Source: CAD feature listing. Evaluate the final solid. Frame: model axes, mm. Give positions to 0.01 mm unless a question says otherwise; leave off trailing zeros. Loops run counter-clockwise (first coordinate to the right, second up) from the corner with the lowest first, then second, coordinate; pieces in that order, holes last. Notation, with made-up numbers: M -35.75,11 L 8.25,11 A25 cw 8.25,47 Z; hole C 54.5,42 d10. An arc over 180 degrees is marked long. Answer in a Markdown table with one row per item.
```python
from build123d import *

# Parameters (mm, degrees)
AUFSATZ_LINEAR_AUSTRAGEN1_DEPTH = 2
AUFSATZ_LINEAR_START            = 2
AUFSATZ_LINEAR_AUSTRAGEN2_DEPTH = 2
SCHNITT_LINEAR_START            = -34
SCHNITT_LINEAR_AUSTRAGEN1_DEPTH = 34
VERRUNDUNG2_START               = 6.1999999
VERRUNDUNG2_3_DEPTH             = 116.6000001


with BuildPart() as part:
    # Skizze1 → Aufsatz-Linear austragen1 (new body)
    with BuildSketch(Plane(origin=(0, 0, 0), x_dir=(1, 0, 0), z_dir=(0, 1, 0))):
        with BuildLine():
            Line((3, 0), (249, 0))
            ThreePointArc((249, 0), (251.121320344, -0.878679656), (252, -3))
            Line((252, -3), (252, -126))
            ThreePointArc((252, -126), (251.121320344, -128.121320344), (249, -129))
            Line((249, -129), (3, -129))
            ThreePointArc((3, -129), (0.878679656, -128.121320344), (0, -126))
            Line((0, -126), (0, -3))
            ThreePointArc((0, -3), (0.878679656, -0.878679656), (3, 0))
        make_face()
        with BuildLine():
            Line((6.2, -3.2), (245.8, -3.2))
            ThreePointArc((245.8, -3.2), (247.921320344, -4.078679656), (248.8, -6.2))
            Line((248.8, -6.2), (248.8, -122.8))
            ThreePointArc((248.8, -122.8), (247.921320344, -124.921320344), (245.8, -125.8))
            Line((245.8, -125.8), (6.2, -125.8))
            ThreePointArc((6.2, -125.8), (4.078679656, -124.921320344), (3.2, -122.8))
            Line((3.2, -122.8), (3.2, -6.2))
            ThreePointArc((3.2, -6.2), (4.078679656, -4.078679656), (6.2, -3.2))
        make_face(mode=Mode.SUBTRACT)
    extrude(amount=AUFSATZ_LINEAR_AUSTRAGEN1_DEPTH)

    # Skizze2 → Aufsatz-Linear austragen2 (add)
    with BuildSketch(Plane.XZ.offset(AUFSATZ_LINEAR_START)):
        with BuildLine():
            Line((6.2, 126.8), (245.8, 126.8))
            ThreePointArc((245.8, 126.8), (248.628427125, 125.628427125), (249.8, 122.8))
            Line((249.8, 122.8), (249.8, 6.2))
            ThreePointArc((249.8, 6.2), (248.628427125, 3.371572875), (245.8, 2.2))
            Line((245.8, 2.2), (6.2, 2.2))
            ThreePointArc((6.2, 2.2), (3.371572875, 3.371572875), (2.2, 6.2))
            Line((2.2, 6.2), (2.2, 122.8))
            ThreePointArc((2.2, 122.8), (3.371572875, 125.628427125), (6.2, 126.8))
        make_face()
        with BuildLine():
            Line((248.8, 122.8), (248.8, 6.2))
            ThreePointArc((248.8, 6.2), (247.921320344, 4.078679656), (245.8, 3.2))
            Line((245.8, 3.2), (6.2, 3.2))
            ThreePointArc((6.2, 3.2), (4.078679656, 4.078679656), (3.2, 6.2))
            Line((3.2, 6.2), (3.2, 122.8))
            ThreePointArc((3.2, 122.8), (4.078679656, 124.921320344), (6.2, 125.8))
            Line((6.2, 125.8), (245.8, 125.8))
            ThreePointArc((245.8, 125.8), (247.921320344, 124.921320344), (248.8, 122.8))
        make_face(mode=Mode.SUBTRACT)
    extrude(amount=-AUFSATZ_LINEAR_AUSTRAGEN2_DEPTH)

    # Skizze3 → Schnitt-Linear austragen1 (cut)
    with BuildSketch(Plane(origin=(0, 2, 0), x_dir=(1, 0, 0), z_dir=(0, 1, 0)).offset(SCHNITT_LINEAR_START)):
        with BuildLine():
            Line((249, 0), (3, 0))
            ThreePointArc((3, 0), (0.878679656, -0.878679656), (0, -3))
            Line((0, -3), (0, -126))
            ThreePointArc((0, -126), (0.878679656, -128.121320344), (3, -129))
            Line((3, -129), (249, -129))
            ThreePointArc((249, -129), (251.121320344, -128.121320344), (252, -126))
            Line((252, -126), (252, -3))
            ThreePointArc((252, -3), (251.121320344, -0.878679656), (249, 0))
        make_face()
        with BuildLine():
            Line((249, -0.2), (3, -0.2))
            ThreePointArc((3, -0.2), (1.020101013, -1.020101013), (0.2, -3))
            Line((0.2, -3), (0.2, -126))
            ThreePointArc((0.2, -126), (1.020101013, -127.979898987), (3, -128.8))
            Line((3, -128.8), (249, -128.8))
            ThreePointArc((249, -128.8), (250.979898987, -127.979898987), (251.8, -126))
            Line((251.8, -126), (251.8, -3))
            ThreePointArc((251.8, -3), (250.979898987, -1.020101013), (249, -0.2))
        make_face(mode=Mode.SUBTRACT)
    extrude(amount=SCHNITT_LINEAR_AUSTRAGEN1_DEPTH, mode=Mode.SUBTRACT)

    # Verrundung2: read off the stored shape, not the designer's step
    # Verrundung2 outline → Verrundung2 (revolve, cut)
    with BuildSketch(Plane(origin=(245.8, 0, 122.8), x_dir=(1, 0, 0), z_dir=(0, 0, 1))):
        with BuildLine():
            Line((3, 2), (3, 1))
            ThreePointArc((3, 1), (3.292893219, 1.707106781), (4, 2))
            Line((4, 2), (3, 2))
        make_face()
    revolve(axis=Axis((245.8, 0, 122.8), (0, 1, 0)), mode=Mode.SUBTRACT)

    # Verrundung2 2 outline → Verrundung2 2 (revolve, cut)
    with BuildSketch(Plane(origin=(245.8, 0, 6.2), x_dir=(1, 0, 0), z_dir=(0, 0, 1))):
        with BuildLine():
            Line((3, 2), (3, 1))
            ThreePointArc((3, 1), (3.292893219, 1.707106781), (4, 2))
            Line((4, 2), (3, 2))
        make_face()
    revolve(axis=Axis((245.8, 0, 6.2), (0, 1, 0)), mode=Mode.SUBTRACT)

    # Verrundung2 3 outline → Verrundung2 3 (cut)
    with BuildSketch(Plane.XY.offset(VERRUNDUNG2_START)):
        with BuildLine():
            ThreePointArc((248.8, 1), (249.092893219, 1.707106781), (249.8, 2))
            Line((249.8, 2), (248.8, 2))
            Line((248.8, 2), (248.8, 1))
        make_face()
    extrude(amount=VERRUNDUNG2_3_DEPTH, mode=Mode.SUBTRACT)


solid = part.part
```
1) Pin query (flat end, axial travel): pin 1 Ø2 at (x, y) = (44, -1.5) entering from +Z. Return the tip coordinate at first contact, or that it passes through.
Reply:
| item | result |
|---|---|
| pin 1 | stops at z = 126.8 |
2) Section B-B, the plane z = 14. Return loops of the section in (x, y), then the cut area to 3 significant figures.
Reply:
| item | result |
|---|---|
| outline | M 0.2,0 L 2.2,0 L 2.2,-2 L 3.2,-2 L 3.2,2 L 0.2,2 Z; M 248.8,-2 L 249.8,-2 L 249.8,0 L 251.8,0 L 251.8,2 L 249.8,2 A1 ccw 248.8,1 Z |
| area | 15.8 mm² |
3) Material intervals for L1, parallel to X at y = -1.2, z = 13; L2, parallel to X at y = 0.5, z = 35; L3, parallel to Z at x = 152.5, y = -1.6, sorted ascending.
Reply:
| item | result |
|---|---|
| L1 | x = 2.2 to 3.2, 248.8 to 249.8 |
| L2 | x = 0.2 to 3.2, 248.8 to 251.8 |
| L3 | z = 2.2 to 3.2, 125.8 to 126.8 |
4) Section A-A, the plane x = 129.5. Return loops of the section in (y, z), then the cut area to 3 significant figures.
Reply:
| item | result |
|---|---|
| outline | M -2,2.2 L 0,2.2 L 0,0.2 L 2,0.2 L 2,3.2 L -2,3.2 Z; M -2,125.8 L 2,125.8 L 2,128.8 L 0,128.8 L 0,126.8 L -2,126.8 Z |
| area | 16.0 mm² |
5) Section C-C, the plane y = -0.85. Return loops of the section in (x, z), then the cut area to 3 significant figures.
Reply:
| item | result |
|---|---|
| outline | M 2.2,6.2 A4 ccw 6.2,2.2 L 245.8,2.2 A4 ccw 249.8,6.2 L 249.8,122.8 A4 ccw 245.8,126.8 L 6.2,126.8 A4 ccw 2.2,122.8 Z; hole M 3.2,6.2 A3 ccw 6.2,3.2 L 245.8,3.2 A3 ccw 248.8,6.2 L 248.8,122.8 A3 ccw 245.8,125.8 L 6.2,125.8 A3 ccw 3.2,122.8 Z |
| area | 734 mm² |
